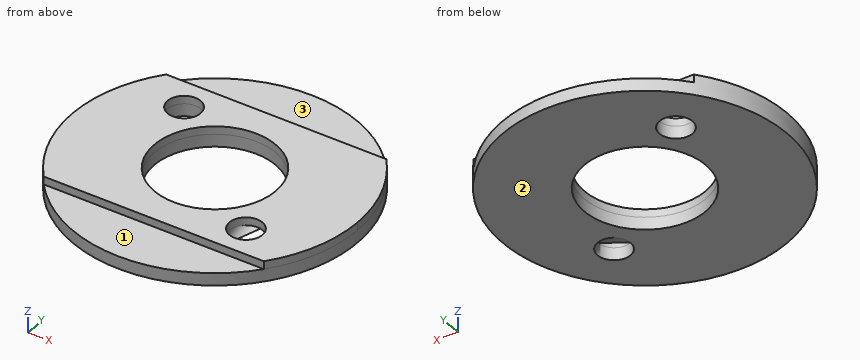
from build123d import *
from build123d.topology import SkipClean

# Parameters (mm, degrees)
SKETCH1_R           = 3.3
SKETCH1_R_2         = 12.15
BOSS_EXTRUDE1_DEPTH = 1.5875
BOSS_EXTRUDE2_START = 2.5
SKETCH2_R           = 28.5
SKETCH2_R_2         = 3.3
SKETCH2_R_3         = 12.15
BOSS_EXTRUDE2_DEPTH = 2.5


with BuildPart() as part:
    # Sketch1 → Boss-Extrude1 (new body)
    with BuildSketch(Plane.XY):
        with BuildLine():
            Line((-4.652672523, -60.083596209), (-48.763782235, -60.083596209))
            ThreePointArc((-48.763782235, -60.083596209), (-55.208227379, -78.133596209), (-48.763782235, -96.183596209))
            Line((-48.763782235, -96.183596209), (-4.652672523, -96.183596209))
            ThreePointArc((-4.652672523, -96.183596209), (0.132351167, -87.716567737), (1.791772621, -78.133596209))
            ThreePointArc((1.791772621, -78.133596209), (0.132351167, -68.550624681), (-4.652672523, -60.083596209))
        make_face()
        with Locations((-12.47433561, -89.950800833)):
            Circle(SKETCH1_R, mode=Mode.SUBTRACT)
        with Locations((-26.708227379, -78.133596209)):
            Circle(SKETCH1_R_2, mode=Mode.SUBTRACT)
        with Locations((-40.942119147, -66.316391585)):
            Circle(SKETCH1_R, mode=Mode.SUBTRACT)
    extrude(amount=BOSS_EXTRUDE1_DEPTH)

    # Sketch2 → Boss-Extrude2 (add)
    with SkipClean():  # the faces are left unmerged after this step: merging them gives an invalid solid
        with BuildSketch(Plane(origin=(0, 0, 0), x_dir=(-1, 0, 0), z_dir=(0, 0, -1)).offset(BOSS_EXTRUDE2_START)):
            with Locations((26.708227379, -78.133596209)):
                Circle(SKETCH2_R)
            with Locations((40.942119147, -66.316391585)):
                Circle(SKETCH2_R_2, mode=Mode.SUBTRACT)
            with Locations((12.47433561, -89.950800833)):
                Circle(SKETCH2_R_2, mode=Mode.SUBTRACT)
            with Locations((26.708227379, -78.133596209)):
                Circle(SKETCH2_R_3, mode=Mode.SUBTRACT)
        extrude(amount=-BOSS_EXTRUDE2_DEPTH)


solid = part.part
The model under review builds one solid part; all positions refer to its coordinate system, in mm. Face numbers are marked on the shaded views. A direction names the side the tool comes from. Round coordinates to 2 decimals unless told otherwise and drop trailing zeros. Write each loop counter-clockwise with the first axis right and the second up, starting at its lowest first coordinate (ties: lowest second). Pieces come first, ordered by that corner, then holes. Notation, with made-up numbers: M -24,6 L 21,6 A16 ccw 21,14 Z; hole C -32.5,84.25 d9. An arc over 180 degrees is marked long. Use a Markdown table: item, result. Add a question column.
Q1. We need section B-B, the plane y = -65. State the section outline as (x, z) points, plus the area to 3 significant figures.
Q2. To check wall thickness, follow line 1 (X direction, y = -78.5, z = -1.35); line 2 (Z direction, x = -44, y = -58); line 3 (Y direction, x = -28, z = -0.45). State the ranges of each line that lie inside material, in increasing order.
Q3. We need section D-D, the plane x = -18.5. State the section outline as (y, z) points.
Q4. Machinability: for the marked faces 1, 2 and 3, which of the approach directions +Z, -Z, +X, -X, +Y, -Y give a long, thin tool a straight path to every point of the face, cutting with its end or side? Answer none if there is none.
Q5. Insertion check: pin 1 (3 mm diameter, centred on x = -31.5, y = -53.5, fed in from +Z); pin 2 (2 mm diameter, centred on x = -8, z = 0.5, fed in from -Y); pin 3 (10 mm diameter, centred on x = -40, y = -64, fed in from +Z); pin 4 (19.5 mm diameter, centred on x = -26.71, y = -78.13, fed in from +Z). Each pin has a flat end and moves straight along its axis. Give the tip position at first contact, or say it passes through.
Findings below:
| question | item | result |
|---|---|---|
| 1 | outline | M -52,-2.5 L -43.97,-2.5 L -43.97,1.59 L -52,1.59 Z; M -37.92,-2.5 L -1.41,-2.5 L -1.41,1.59 L -37.92,1.59 Z |
| 1 | area | 182 mm² |
| 2 | line 1 | x = -55.21 to -38.85, -14.56 to 1.79 |
| 2 | line 2 | z = -2.5 to 0 |
| 2 | line 3 | y = -106.6 to -90.21, -66.05 to -49.66 |
| 3 | outline | M -105.43,-2.5 L -87.09,-2.5 L -87.09,1.59 L -96.18,1.59 L -96.18,0 L -105.43,0 Z; M -69.18,-2.5 L -50.84,-2.5 L -50.84,0 L -60.08,0 L -60.08,1.59 L -69.18,1.59 Z |
| 4 | face 1 | +Z, +X, -X, -Y |
| 4 | face 2 | -Z, +X, -X, +Y, -Y |
| 4 | face 3 | +Z, +X, -X, +Y |
| 5 | pin 1 | stops at z = 0 |
| 5 | pin 2 | stops at y = -100.36 |
| 5 | pin 3 | stops at z = 1.59 |
| 5 | pin 4 | passes through |
